The listing builds one solid part. Answer for the finished solid, in the listing's coordinates (mm). A direction names the side the tool comes from. Coordinates: 2 decimals unless noted, no trailing zeros. Order: outer loops, then holes, each group sorted by start corner. A loop starts at its lowest first (then second) coordinate and runs counter-clockwise, first axis right, second up. Notation, with made-up numbers: (-32.5, 40) -> (23.5, 40) arc R31 cw to (23.5, 78) -> close; hole circle Ø11 at (37.5, 83.5). An arc over 180 degrees is marked (long way). Answer in a Markdown table with one row per item.
Autodesk Inventor part; units mm, degrees
ref_plane "YZ Plane" through (0, 0, 0) normal (1, 0, 0) x (0, 1, 0)
ref_plane "XZ Plane" through (0, 0, 0) normal (0, 1, 0) x (-1, 0, 0)
ref_plane "XY Plane" through (0, 0, 0) normal (0, 0, 1) x (1, 0, 0)
sketch "Sketch1" plane through (0, 0, 0) normal (1, 0, 0) x (0, 1, 0)
  line L0 (0, 0) -> (25.4, 0)
  line L1 (25.4, 0) -> (25.4, -9.525)
  line L2 (25.4, -9.525) -> (0, -9.525)
  line L3 (0, -9.525) -> (0, 0)
  dimension "d0" = 25.4
  dimension "d1" = 9.525
extrude "Extrusion1" add sketch "Sketch1" along normal blind 6.35
sketch "Sketch2" plane through (6.35, 0, 0) normal (1, 0, 0) x (0, 0, -1)
  line L0 (9.525, 25.4) -> (0, 25.4)
  line L1 (0, 0) -> (9.525, 25.4)
  line L2 (9.525, 25.4) -> (0, 25.4)
  line L3 (0, 0) -> (9.525, 0)
  line L4 (0, 25.4) -> (9.525, 0)
  circle A0 centre (4.7625, 12.7) radius 9.779
  circle A1 centre (4.7625, 22.479) radius 1.7907
  circle A2 centre (4.7625, 2.921) radius 1.7907
  dimension "d4" = 19.558
  dimension "d5" = 3.5814
  dimension "d6" = 3.5814
extrude "Extrusion2" cut sketch "Sketch2" against normal blind 14.2875 contours A1 A0 | A0 A1 | A2 A0 | A0 A2
sketch "Sketch3" plane through (6.35, 0, 0) normal (1, 0, 0) x (0, 0, -1)
  line L0 (9.525, 25.4) -> (0, 25.4)
  arc A0 (9.525, 25.4) -> (0, 25.4) centre (4.7625, 24.3714) ccw
  point P0 (0, 0)
extrude "Extrusion3" add sketch "Sketch3" against normal blind 6.35
sketch "Sketch4" plane through (6.35, 0, 0) normal (1, 0, 0) x (0, 0, -1)
  line L0 (0, 0) -> (9.525, 0)
  line L1 (9.525, 0) -> (0, 0)
  line L2 (0, 0) -> (0, -25.4)
  line L3 (0, -25.4) -> (9.525, -25.4)
  line L4 (9.525, -25.4) -> (9.525, 0)
  dimension "d15" = 25.4
extrude "Extrusion4" add sketch "Sketch4" against normal blind 6.35
sketch "Sketch5" plane through (6.35, 0, 0) normal (1, 0, 0) x (0, 0, -1)
  line L0 (9.525, -25.4) -> (9.525, 25.4)
  line L1 (9.525, -9.7563) -> (33.5033, -25.4)
  line L2 (33.5033, -25.4) -> (9.525, -25.4)
  point P0 (0, 0)
extrude "Extrusion5" add sketch "Sketch5" against normal blind 6.35
sketch "Sketch6" plane through (6.35, 0, 0) normal (1, 0, 0) x (0, 0, -1)
  line L0 (26.3764, -37.8164) -> (39.194, -37.8164)
  line L1 (39.194, -37.8164) -> (39.194, -17.7508)
  line L2 (39.194, -17.7508) -> (26.3764, -17.7508)
  line L3 (26.3764, -17.7508) -> (26.3764, -37.8164)
  point P0 (0, 0)
extrude "Extrusion6" cut sketch "Sketch6" against normal blind 63.5
properties part number "GripperOnS"
(1) A cutting plane is placed at B-B, the plane x = 4.5. Determine the outline of the cut face in (y, z) (1 decimal), then the cut area to 3 significant figures.
Check values:
| item | result |
|---|---|
| outline | (-25.4, -26.4) -> (-20.8, -26.4) -> (-9.8, -9.5) -> (25.4, -9.5) arc R4.9 ccw to (25.4, 0) -> (-25.4, 0) -> close; hole circle Ø3.6 at (2.9, -4.8); hole circle Ø3.6 at (22.5, -4.8) |
| area | 662 mm² |
(2) Flat-ended cylindrical pins translate along their axes: pin 1 (3 mm diameter, centred on y = 22.48, z = -4.76, fed in from -X); pin 2 (1 mm diameter, centred on x = 2.5, y = 4.5, fed in from -Z) (3 decimals). Find the tip coordinate at first contact, or state that the pin passes through.
Check values:
| item | result |
|---|---|
| pin 1 | through |
| pin 2 | z = -9.525 |
(3) Which of the six approach directions +Z, -Z, +X, -X, +Y, -Y give full straight-line access (tool end or side, diameter ignored) to faces 4 (the flat face through (3, -23, -26.376)), 5 (the flat face through (3, 8, -9.525))?
Check values:
| item | result |
|---|---|
| face 4 | -Z, +X, -X, +Y, -Y |
| face 5 | -Z, +X, -X, +Y |
(4) For a pull along Y with two mould halves and no side action, classify faces 1 (the cylindrical face through (3.219, 1.831, -3.341)), 2 (the flat face through (0, -4, -7)), 3 (the flat face through (3, -25.4, -13)) as released by +Y, released by -Y, zero draft, split by the parting line, or undercut.
Check values:
| item | result |
|---|---|
| face 1 | undercut |
| face 2 | zero draft |
| face 3 | released by -Y |
(5) Find the intervals of material crossed by line 1 along Y through (x, z) = (0.5, -3.5); line 2 along Z through (x, y) = (5.25, 3) (3 decimals); line 3 along Z through (x, y) = (4.25, -8.5) (3 decimals), in increasing order. Write a range as from..to.
Check values:
| item | result |
|---|---|
| line 1 | -25.4..1.65, 4.19..21.21, 23.75..29.08 |
| line 2 | -9.525..-6.551, -2.974..0 |
| line 3 | -9.525..0 |
(6) A cutting plane is placed at A-A, the plane z = -5.75. Determine the outline of the cut face in (x, y), then the cut area to 3 significant figures.
Check values:
| item | result |
|---|---|
| outline | (0, -25.4) -> (6.35, -25.4) -> (6.35, 1.43) -> (0, 1.43) -> close; (0, 4.41) -> (6.35, 4.41) -> (6.35, 20.99) -> (0, 20.99) -> close; (0, 23.97) -> (6.35, 23.97) -> (6.35, 29.14) -> (0, 29.14) -> close |
| area | 308 mm² |
(7) A cutting plane is placed at D-D, the plane z = -19.5. Determine the outline of the cut face in (x, y), then the cut area to 3 significant figures.
Check values:
| item | result |
|---|---|
| outline | (0, -25.4) -> (6.35, -25.4) -> (6.35, -16.26) -> (0, -16.26) -> close |
| area | 58.0 mm² |
(8) A cutting plane is placed at C-C, the plane y = 15. Determine the outline of the cut face in (x, z) (3 decimals).
Check values:
| item | result |
|---|---|
| outline | (0, -9.525) -> (6.35, -9.525) -> (6.35, 0) -> (0, 0) -> close |
